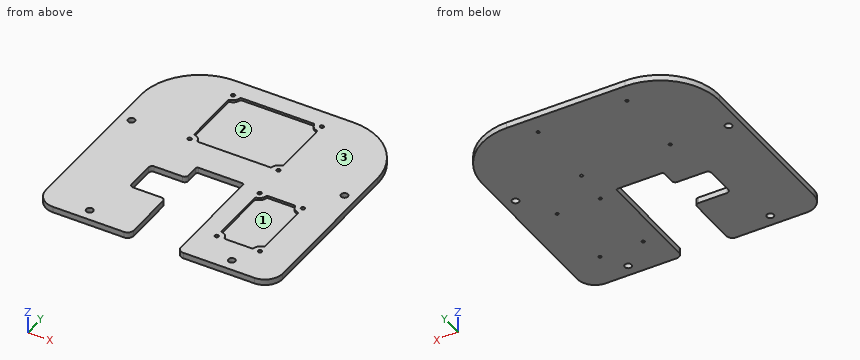
from build123d import *

# Parameters (mm, degrees)
SKETCH_1_W          = 200
SKETCH_1_H          = 200
EXTRUDE_1_DEPTH     = 5
SKETCH_2_W          = 40
SKETCH_2_H          = 95
CUT_EXTRUDE_1_DEPTH = 149.744747806
FILLET_1_R          = 50
FILLET_2_R          = 1.5
SKETCH_3_W          = 30
SKETCH_3_H          = 30
CUT_EXTRUDE_2_DEPTH = 10
FILLET_3_R          = 3
M3X0_5_2_D          = 2.5
M3X0_5_1_D          = 2.5
FILLET_4_R          = 15
FILLET_5_R          = 5
HOLE_WIZARD_M5_1_D  = 5.8
SKETCH_4_R          = 1.6
CUT_EXTRUDE_3_DEPTH = 2
SKETCH_7_R          = 1.6
CUT_EXTRUDE_4_DEPTH = 2


with BuildPart() as part:
    # ｽｹｯﾁ1 → ﾎﾞｽ - 押し出し1 (new body)
    with BuildSketch(Plane.XY):
        with Locations((0, 10)):
            Rectangle(SKETCH_1_W, SKETCH_1_H)
    extrude(amount=EXTRUDE_1_DEPTH)

    # ｽｹｯﾁ2 → ｶｯﾄ - 押し出し1 (cut, through all)
    with BuildSketch(Plane.XY.offset(5)):
        with Locations((0, -42.5)):
            Rectangle(SKETCH_2_W, SKETCH_2_H)
    extrude(amount=-CUT_EXTRUDE_1_DEPTH, mode=Mode.SUBTRACT)

    # ﾌｨﾚｯﾄ1
    fillet_1_edges = [part.edges().sort_by_distance(p)[0] for p in [
        (-100, 110, 2.5),
        (100, 110, 2.5),
    ]]
    fillet(fillet_1_edges, radius=FILLET_1_R)

    # ﾌｨﾚｯﾄ2
    fillet_2_edges = [part.edges().sort_by_distance(p)[0] for p in [
        (-20, 5, 2.5),
        (20, 5, 2.5),
    ]]
    fillet(fillet_2_edges, radius=FILLET_2_R)

    # ｽｹｯﾁ3 → ｶｯﾄ - 押し出し2 (cut)
    with BuildSketch(Plane(origin=(0, 0, 0), x_dir=(-1, 0, 0), z_dir=(0, 0, -1))):
        with Locations((35, -25)):
            Rectangle(SKETCH_3_W, SKETCH_3_H)
    extrude(amount=-CUT_EXTRUDE_2_DEPTH, mode=Mode.SUBTRACT)

    # ﾌｨﾚｯﾄ3
    fillet_3_edges = [part.edges().sort_by_distance(p)[0] for p in [
        (-20, -40, 2.5),
        (-20, -10, 2.5),
        (-50, -10, 2.5),
        (-50, -40, 2.5),
    ]]
    fillet(fillet_3_edges, radius=FILLET_3_R)

    # M3x0.5 ねじ穴用ねじ下穴ﾄﾞﾘﾙ2 (through all)
    with Locations(Plane.XY.offset(5)):
        with Locations((-42, 94), (33, 94), (-42, 32), (33, 32)):
            Hole(M3X0_5_2_D / 2)

    # M3x0.5 ねじ穴用ねじ下穴ﾄﾞﾘﾙ1 (through all)
    with Locations(Plane.XY.offset(5)):
        with Locations((35.5, 1), (72, 1), (35.5, -60), (72, -60)):
            Hole(M3X0_5_1_D / 2)

    # ﾌｨﾚｯﾄ4
    fillet_4_edges = [part.edges().sort_by_distance(p)[0] for p in [
        (100, -90, 2.5),
        (-100, -90, 2.5),
    ]]
    fillet(fillet_4_edges, radius=FILLET_4_R)

    # ﾌｨﾚｯﾄ5
    fillet_5_edges = [part.edges().sort_by_distance(p)[0] for p in [
        (-20, -90, 2.5),
        (20, -90, 2.5),
    ]]
    fillet(fillet_5_edges, radius=FILLET_5_R)

    # M5 すきま穴1 (through all)
    with Locations(Plane(origin=(0, 0, 0), x_dir=(-1, 0, 0), z_dir=(0, 0, -1))):
        with Locations((-60, -80), (60, -80), (-90, 30), (90, 30)):
            Hole(HOLE_WIZARD_M5_1_D / 2)

    # ｽｹｯﾁ4 → ｶｯﾄ - 押し出し3 (cut)
    with BuildSketch(Plane.XY.offset(5)):
        with Locations((-42, 94)):
            Circle(SKETCH_4_R)
        with Locations((33, 94)):
            Circle(SKETCH_4_R)
        with Locations((-42, 32)):
            Circle(SKETCH_4_R)
        with Locations((33, 32)):
            Circle(SKETCH_4_R)
        with BuildLine():
            Line((-34.651530772, 94), (25.651530772, 94))
            ThreePointArc((25.651530772, 94), (26.60021407, 93.661895004), (27.121224617, 92.8))
            ThreePointArc((27.121224617, 92.8), (28.757359313, 89.757359313), (31.8, 88.121224617))
            ThreePointArc((31.8, 88.121224617), (32.661895004, 87.60021407), (33, 86.651530772))
            Line((33, 86.651530772), (33, 39.348469228))
            ThreePointArc((33, 39.348469228), (32.661895004, 38.39978593), (31.8, 37.878775383))
            ThreePointArc((31.8, 37.878775383), (28.757359313, 36.242640687), (27.121224617, 33.2))
            ThreePointArc((27.121224617, 33.2), (26.60021407, 32.338104996), (25.651530772, 32))
            Line((25.651530772, 32), (-34.651530772, 32))
            ThreePointArc((-34.651530772, 32), (-35.60021407, 32.338104996), (-36.121224617, 33.2))
            ThreePointArc((-36.121224617, 33.2), (-37.757359313, 36.242640687), (-40.8, 37.878775383))
            ThreePointArc((-40.8, 37.878775383), (-41.661895004, 38.39978593), (-42, 39.348469228))
            Line((-42, 39.348469228), (-42, 86.651530772))
            ThreePointArc((-42, 86.651530772), (-41.661895004, 87.60021407), (-40.8, 88.121224617))
            ThreePointArc((-40.8, 88.121224617), (-37.757359313, 89.757359313), (-36.121224617, 92.8))
            ThreePointArc((-36.121224617, 92.8), (-35.60021407, 93.661895004), (-34.651530772, 94))
        make_face()
    extrude(amount=-CUT_EXTRUDE_3_DEPTH, mode=Mode.SUBTRACT)

    # ｽｹｯﾁ7 → ｶｯﾄ - 押し出し4 (cut)
    with BuildSketch(Plane.XY.offset(5)):
        with Locations((35.5, 1)):
            Circle(SKETCH_7_R)
        with Locations((72, 1)):
            Circle(SKETCH_7_R)
        with Locations((35.5, -60)):
            Circle(SKETCH_7_R)
        with Locations((72, -60)):
            Circle(SKETCH_7_R)
        with BuildLine():
            Line((64.651530772, -60), (42.848469228, -60))
            ThreePointArc((42.848469228, -60), (41.89978593, -59.661895004), (41.378775383, -58.8))
            ThreePointArc((41.378775383, -58.8), (39.742640687, -55.757359313), (36.7, -54.121224617))
            ThreePointArc((36.7, -54.121224617), (35.838104996, -53.60021407), (35.5, -52.651530772))
            Line((35.5, -52.651530772), (35.5, -6.348469228))
            ThreePointArc((35.5, -6.348469228), (35.838104996, -5.39978593), (36.7, -4.878775383))
            ThreePointArc((36.7, -4.878775383), (39.742640687, -3.242640687), (41.378775383, -0.2))
            ThreePointArc((41.378775383, -0.2), (41.89978593, 0.661895004), (42.848469228, 1))
            Line((42.848469228, 1), (64.651530772, 1))
            ThreePointArc((64.651530772, 1), (65.60021407, 0.661895004), (66.121224617, -0.2))
            ThreePointArc((66.121224617, -0.2), (67.757359313, -3.242640687), (70.8, -4.878775383))
            ThreePointArc((70.8, -4.878775383), (71.661895004, -5.39978593), (72, -6.348469228))
            Line((72, -6.348469228), (72, -52.651530772))
            ThreePointArc((72, -52.651530772), (71.661895004, -53.60021407), (70.8, -54.121224617))
            ThreePointArc((70.8, -54.121224617), (67.757359313, -55.757359313), (66.121224617, -58.8))
            ThreePointArc((66.121224617, -58.8), (65.60021407, -59.661895004), (64.651530772, -60))
        make_face()
    extrude(amount=-CUT_EXTRUDE_4_DEPTH, mode=Mode.SUBTRACT)


solid = part.part
Check sheet for the modelled part. Datum: model origin and axes. Units: mm. Face numbers are marked on the shaded views. Coordinates: 2 decimals unless noted, no trailing zeros. Loops run counter-clockwise (first coordinate to the right, second up) from the corner with the lowest first, then second, coordinate; pieces in that order, holes last. Notation, with made-up numbers: (73, 88) -> (80, 88) arc R28 cw to (80, 111) -> close; hole circle Ø1 at (-19, 18.5). An arc over 180 degrees is marked (long way). Write item = value, one per line. Start each with the question number.
1. Section check B-B on x = -90. Record the cut outline in (y, z), then the cut area to 3 significant figures.
2. Section check D-D on z = 2.15. Give the number of separate pieces and of enclosed holes in the cut face, then the cut area to 3 significant figures.
3. Draft check along X on the marked faces 1, 2 and 3. Enter one of: released by +X, released by -X, zero draft, split by the parting line, or undercut.
4. Section check A-A on y = -71. Record the cut outline in (x, z).
5. Section check C-C on y = 74. Record the cut outline in (x, z).
6. Material ranges on line 1 (Y direction, x = 33, z = 0.9); line 2 (Y direction, x = -3.5, z = 3.9); line 3 (Y direction, x = 72, z = 1.45), recorded low to high.
7. Depth check by flat-ended pin: P1, Ø1, axis at x = 80, z = 1, coming from the +Y side; P2, Ø1, axis at x = -13.5, z = 4.5, coming from the -Y side; P3, Ø3, axis at x = 35.5, y = -60, coming from the +Z side; P4, Ø1.5, axis at x = -42, y = 32, coming from the +Z side. Enter the tip coordinate at first touch or a pass-through.
Responses:
q1.outline = (-89.14, 0) -> (27.1, 0) -> (27.1, 5) -> (-89.14, 5) -> close; (32.9, 0) -> (90, 0) -> (90, 5) -> (32.9, 5) -> close
q1.area = 867 mm2
q2.separate_pieces = 1
q2.enclosed_holes = 12
q2.area = 34,000 mm2
q3.face_1 = undercut
q3.face_2 = undercut
q3.face_3 = zero draft
q4.outline = (-100, 0) -> (-20, 0) -> (-20, 5) -> (-100, 5) -> close; (20, 0) -> (100, 0) -> (100, 5) -> (20, 5) -> close
q5.outline = (-98, 0) -> (98, 0) -> (98, 5) -> (33, 5) -> (33, 3) -> (-42, 3) -> (-42, 5) -> (-98, 5) -> close
q6.line_1 = -90 to 30.75, 33.25 to 92.75, 95.25 to 110
q6.line_2 = 5 to 32, 94 to 110
q6.line_3 = -90 to -61.25, -58.75 to -0.25, 2.25 to 104.9
q7.P1 = 100.37
q7.P2 = 5
q7.P3 = 3
q7.P4 = through
